Model file for the job. Use its own axes, mm. A direction names the side the tool comes from. Round coordinates to 2 decimals unless told otherwise and drop trailing zeros. Loops run counter-clockwise (first coordinate to the right, second up) from the corner with the lowest first, then second, coordinate; pieces in that order, holes last. Notation, with made-up numbers: (53, 61.25) - (81, 61.25) arc R24 cw to (81, 99.25) - close; hole circle Ø1 at (4, 78.5). An arc over 180 degrees is marked (long way). Use one line per item in the form item = value.
from build123d import *

# Parameters (mm, degrees)
BOSS_EXTRUDE1_DEPTH          = 24
SKETCH2_W                    = 30.110806601
SKETCH2_H                    = 12
CUT_EXTRUDE1_DEPTH           = 45.271887242
CUT_EXTRUDE2_DEPTH           = 6.8
F_7_8_8_DIAMETER_HOLE1_D     = 8
F_7_8_8_DIAMETER_HOLE1_DEPTH = 6.2
F_7_8_8_DIAMETER_HOLE2_D     = 8
F_4_7_5_DIAMETER_HOLE2_D     = 5
F_4_7_5_DIAMETER_HOLE2_DEPTH = 6
F_4_7_5_DIAMETER_HOLE1_D     = 5


with BuildPart() as part:
    # Sketch1 → Boss-Extrude1 (new body)
    with BuildSketch(Plane(origin=(0, 0, -24), x_dir=(-1, 0, 0), z_dir=(0, 0, -1))):
        with BuildLine():
            Line((0, 11), (-30, 11))
            Line((-30, 11), (-30, -11))
            Line((-30, -11), (0, -11))
            ThreePointArc((0, -11), (11, 0), (0, 11))
        make_face()
    extrude(amount=-BOSS_EXTRUDE1_DEPTH)

    # Sketch2 → Cut-Extrude1 (cut, through all)
    with BuildSketch(Plane(origin=(0, 11, 0), x_dir=(-1, 0, 0), z_dir=(0, 1, 0))):
        with Locations((2.055403301, -12)):
            Rectangle(SKETCH2_W, SKETCH2_H)
    extrude(amount=-CUT_EXTRUDE1_DEPTH, mode=Mode.SUBTRACT)

    # Sketch3 → Cut-Extrude2 (cut)
    with BuildSketch(Plane(origin=(19.2, 0, 0), x_dir=(0, -1, 0), z_dir=(-1, 0, 0))):
        Polygon((11, -18.5), (11, -5.5), (-3.75277675, -5.5), (-7.505553499, -12), (-3.75277675, -18.5), align=None)
    extrude(amount=-CUT_EXTRUDE2_DEPTH, mode=Mode.SUBTRACT)

    # Ø7.8 (8) Diameter Hole1
    with Locations(Plane.ZY.offset(-13)):
        with Locations((-12, 0)):
            Hole(F_7_8_8_DIAMETER_HOLE1_D / 2, depth=F_7_8_8_DIAMETER_HOLE1_DEPTH)

    # Ø7.8 (8) Diameter Hole2 (through all)
    with Locations(Plane.ZY.offset(-26)):
        with Locations((-12, 0)):
            Hole(F_7_8_8_DIAMETER_HOLE2_D / 2)

    # Ø4.7 (5) Diameter Hole2
    with Locations(Plane(origin=(0, 0, -24), x_dir=(-1, 0, 0), z_dir=(0, 0, -1))):
        with Locations((0, 0)):
            Hole(F_4_7_5_DIAMETER_HOLE2_D / 2, depth=F_4_7_5_DIAMETER_HOLE2_DEPTH)

    # Ø4.7 (5) Diameter Hole1 (through all)
    with Locations(Plane(origin=(0, 0, -6), x_dir=(-1, 0, 0), z_dir=(0, 0, -1))):
        with Locations((0, 0)):
            Hole(F_4_7_5_DIAMETER_HOLE1_D / 2)


solid = part.part
1. Cut at D-D, the plane x = -1.5. Give the cut face in (y, z), plus the area to 3 significant figures.
Geometry check:
outline = (-10.9, -24) - (-2, -24) - (-2, -18) - (-10.9, -18) - close; (-10.9, -6) - (-2, -6) - (-2, 0) - (-10.9, 0) - close; (2, -24) - (10.9, -24) - (10.9, -18) - (2, -18) - close; (2, -6) - (10.9, -6) - (10.9, 0) - (2, 0) - close
area = 214 mm^2
2. Pull direction X, two halves, no side cores. Call faces 1 (the flat face through (15, -11, -12)), 2 (the cylindrical face through (-11, 0, -3)), 3 (the cylindrical face through (-0.54, -2.44, -20.96)): +X half, -X half, draft (parallel to the pull), parting line (faces both ways), or undercut.
Geometry check:
face_1 = draft
face_2 = -X half
face_3 = undercut
3. Wall check: probe 1 along Z at (x, y) = (-4.5, 8); probe 2 along X at (y, z) = (-9.25, -14); probe 3 along Y at (x, z) = (16, -12). Give the ranges that are in metal, low to high.
Geometry check:
probe_1 = -24 to -18, -6 to 0
probe_2 = 13 to 19.2, 26 to 30
probe_3 = -11 to -4, 4 to 11
4. Cut at A-A, the plane y = 0. Give the cut face in (x, z), plus the area to 3 significant figures.
Geometry check:
outline = (-11, -24) - (-2.5, -24) - (-2.5, -18) - (-11, -18) - close; (-11, -6) - (-2.5, -6) - (-2.5, 0) - (-11, 0) - close; (2.5, -24) - (30, -24) - (30, -16) - (26, -16) - (26, -18.5) - (19.2, -18.5) - (19.2, -16) - (13, -16) - (13, -18) - (2.5, -18) - close; (2.5, -6) - (13, -6) - (13, -8) - (19.2, -8) - (19.2, -5.5) - (26, -5.5) - (26, -8) - (30, -8) - (30, 0) - (2.5, 0) - close
area = 466 mm^2
5. Tool access for faces 4 (the flat face through (22.6, 5.6, -8.7)), 5 (the flat face through (18, 11, -12)), 6 (the flat face through (4, 0, -6)): list every direction of +Z, -Z, +X, -X, +Y, -Y with a clear straight run to the whole face (end or side of a thin tool).
Geometry check:
face_4 = -Y
face_5 = +Z, -Z, +X, -X, +Y
face_6 = -X, +Y, -Y
6. Cut at C-C, the plane z = -22. Give the cut face in (x, y).
Geometry check:
outline = (0, -11) - (30, -11) - (30, 11) - (0, 11) arc R11 ccw to start; hole circle Ø5 at (0, 0)
7. Cut at B-B, the plane x = 16. Give the cut face in (y, z).
Geometry check:
outline = (-11, -24) - (11, -24) - (11, 0) - (-11, 0) - close; hole circle Ø8 at (0, -12)
8. Flat gauge pins, fed straight in: pin 1 (3.5 mm diameter, centred on y = -3, z = -10.5, fed in from -X); pin 2 (4 mm diameter, centred on x = 0, y = 0, fed in from -Z); pin 3 (3 mm diameter, centred on y = 2.5, z = -19.5, fed in from -X). Where does each tip first touch, or does it go through?
Geometry check:
pin_1 = 13
pin_2 = through
pin_3 = -10.95
